Source: CAD feature listing. Evaluate the final solid. Frame: model axes, mm. Face numbers are marked on the shaded views. A direction names the side the tool comes from. Give positions to 0.01 mm unless a question says otherwise; leave off trailing zeros. Order: outer loops, then holes, each group sorted by start corner. A loop starts at its lowest first (then second) coordinate and runs counter-clockwise, first axis right, second up. Notation, with made-up numbers: (-17, 73) -> (-9, 73) arc R14 ccw to (-9, 94) -> close; hole circle Ø6 at (1.25, 84). An arc over 180 degrees is marked (long way). Answer in a Markdown table with one row per item.
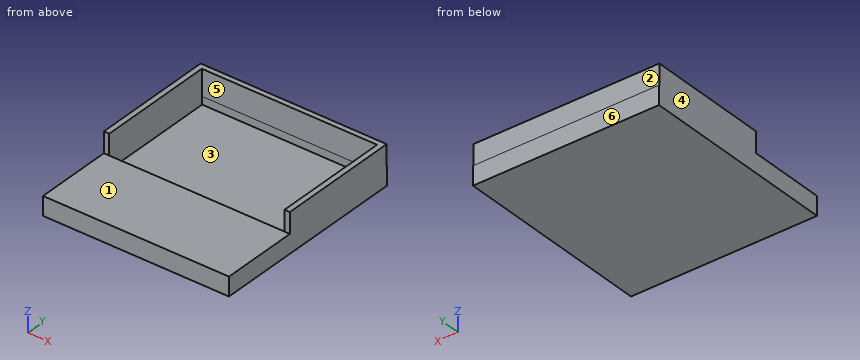
```python
from build123d import *

# Parameters (mm, degrees)
F0_W          = 87
F0_H          = 8.7780428881
F1_DEPTH      = 47
F1_DEPTH_BACK = 47
F2_W          = 57.5710088015
F2_H          = 14.0236988664
F3_DEPTH      = 43.5
F3_DEPTH_BACK = 43.5
F4_T          = 2.5
F4_T3_DEPTH   = 92


# Not quite as in the source:
# - a shell that OpenCascade refuses in one call is made with other operations: the cavity is built on its own and cut out
# - the program builds the solid bodies; features that only make, move or delete a surface that nothing else refers to are left out


with BuildPart() as f1:
    # F0 (on Front) → F1 (new body, two sides)
    with BuildSketch(Plane.XZ) as f1_sk:
        Rectangle(F0_W, F0_H)
    extrude(amount=F1_DEPTH)
    extrude(f1_sk.sketch, amount=-F1_DEPTH_BACK)

    # F2 (on Right) → F3 (join, two sides)
    with BuildSketch(Plane.YZ) as f3_sk:
        with Locations((18.0093571544, 7.0118494332)):
            Rectangle(F2_W, F2_H)
    extrude(amount=F3_DEPTH)
    extrude(f3_sk.sketch, amount=-F3_DEPTH_BACK)

    # F4: shell of thickness 2.5, made by hand


with BuildPart() as f4_core1:
    # F4_t2: copy of F1
    add(f1.part)

    # the walls: a layer under each face that stays
    f4_faces = [f4_core1.faces().sort_by_distance(p)[0] for p in [
        (-43.5, 0, 4.8173387112),
        (0, -28.8880736232, 4.3890214441),
        (0, 46.8974307775, 4.3890214441),
        (0, 47, 0),
        (0, 0, -4.3890214441),
        (0, -47, 0),
        (43.5, 0, 4.8173387112),
        (0, 46.7948615551, 9.2063601552),
    ]]
    thicken(f4_faces, amount=-F4_T, mode=Mode.SUBTRACT)

    # F4_s4 → F4_t3 (cut)
    with BuildSketch(Plane.YZ.offset(-46)):
        Polygon((46.8198615551, 4.4140214441), (46.7948615551, 1.8890214441), (44.2948615551, 1.8890214441), (44.2948615551, 4.3890214441), align=None)
    extrude(amount=F4_T3_DEPTH, mode=Mode.SUBTRACT)


with BuildPart() as f1_1:
    add(f1.part)

    # what is left inside the walls is the cavity
    f4_cavity = [f4_core1.part.solids().sort_by_distance(p)[0] for p in [
        (0, -14.833333, -1.864021),
    ]]
    add(f4_cavity, mode=Mode.SUBTRACT)


solid = f1_1.part
```
(1) Access query for the marked faces 1, 2 and 3. Directions: +Z, -Z, +X, -X, +Y, -Y. A direction counts if a zero-diameter tool reaches every point of the face in a straight line with its end or side. Return the directions, or none.
A:
| item | result |
|---|---|
| face 1 | +Z, +X, -X, -Y |
| face 2 | +Z, +X, -X, +Y |
| face 3 | none |
(2) Ray query, probe 1 along X at (y, z) = (21, 2); probe 2 along Y at (x, z) = (37.5, -1.5); probe 3 along Z at (x, y) = (-32.5, -36). Return the intervals inside material, ascending.
A:
| item | result |
|---|---|
| probe 1 | x = -43.5 to -41, 41 to 43.5 |
| probe 2 | y = -47 to -44.5, 44.5 to 47 |
| probe 3 | z = -4.39 to -1.89, 1.89 to 4.39 |
(3) Pull-direction query (X, two-part tool) for the marked faces 4, 5 and 6; classes: +X half, -X half, draft (parallel to the pull), parting line (faces both ways), or undercut.
A:
| item | result |
|---|---|
| face 4 | -X half |
| face 5 | undercut |
| face 6 | draft |
(4) Section query B-B (z = -0.25). Return the cut outline in (x, y).
A:
| item | result |
|---|---|
| outline | (-43.5, -47) -> (43.5, -47) -> (43.5, 47) -> (-43.5, 47) -> close; hole (-41, -44.5) -> (41, -44.5) -> (41, 44.5) -> (-41, 44.5) -> close |
(5) Section query C-C (x = -20.5). Return the cut outline in (y, z).
A:
| item | result |
|---|---|
| outline | (-47, -4.39) -> (47, -4.39) -> (47, 4.39) -> (46.79, 4.39) -> (46.79, 14.02) -> (44.29, 14.02) -> (44.29, 1.89) -> (44.5, 1.89) -> (44.5, -1.89) -> (-44.5, -1.89) -> (-44.5, 1.89) -> (-10.78, 1.89) -> (-10.78, 4.39) -> (-47, 4.39) -> close |
(6) Section query A-A (y = -40). Return the cut outline in (x, z), plus the area to 3 significant figures.
A:
| item | result |
|---|---|
| outline | (-43.5, -4.39) -> (43.5, -4.39) -> (43.5, 4.39) -> (-43.5, 4.39) -> close; hole (-41, -1.89) -> (41, -1.89) -> (41, 1.89) -> (-41, 1.89) -> close |
| area | 454 mm^2 |
(7) First-contact query: pin 1 Ø9.5 at (x, z) = (4.5, 8) entering from -Y; pin 2 Ø1.5 at (x, y) = (-7.5, 28) entering from +Z; pin 3 Ø1.5 at (x, y) = (15, -25.5) entering from +Z; pin 4 Ø2 at (x, z) = (42, 11) entering from -Y. Flat tips, straight axial feed; report the tip coordinate or a pass-through.
A:
| item | result |
|---|---|
| pin 1 | stops at y = -47 |
| pin 2 | stops at z = -1.89 |
| pin 3 | stops at z = 4.39 |
| pin 4 | stops at y = -10.78 |
(8) Section query D-D (y = 27). Return the cut outline in (x, z), plus the area to 3 significant figures.
A:
| item | result |
|---|---|
| outline | (-43.5, -4.39) -> (43.5, -4.39) -> (43.5, 14.02) -> (41, 14.02) -> (41, -1.89) -> (-41, -1.89) -> (-41, 14.02) -> (-43.5, 14.02) -> close |
| area | 297 mm^2 |
